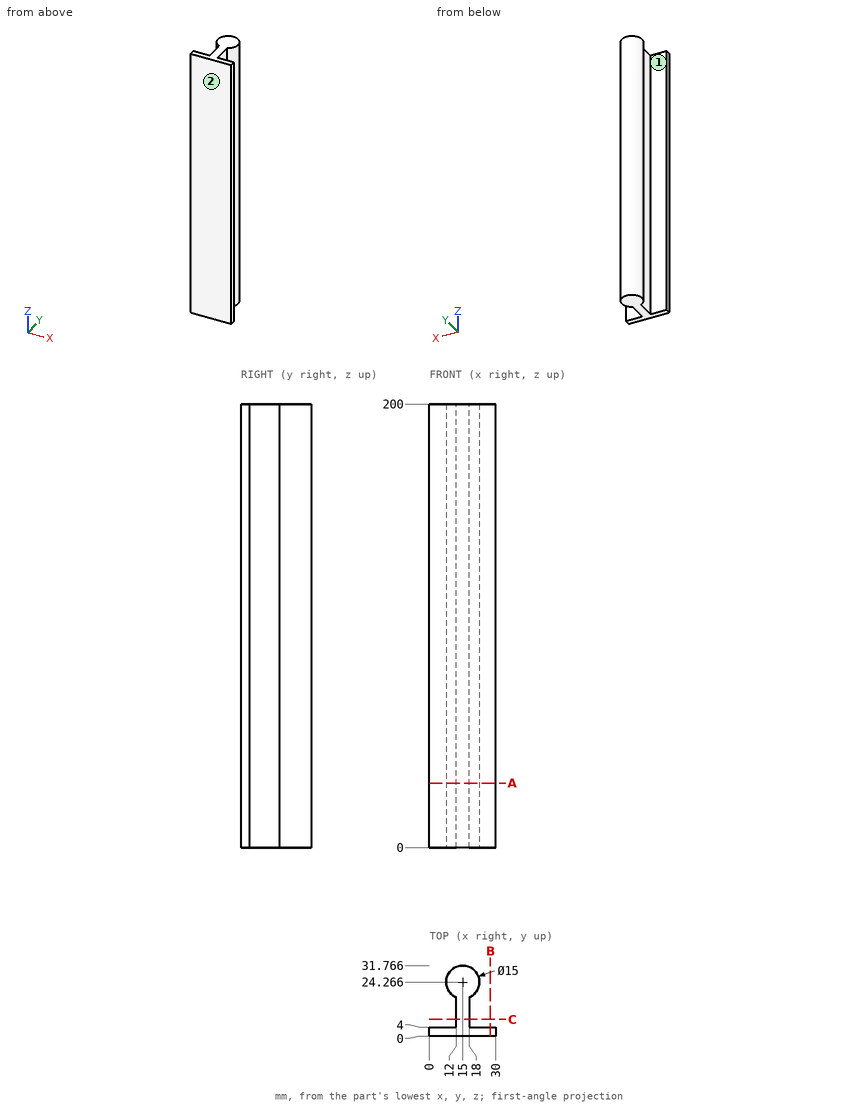
Check sheet for the drawn part. Datum: minimum x, y, z corner. Units: mm. Round coordinates to 2 decimals unless told otherwise and drop trailing zeros. Loops run counter-clockwise (first coordinate to the right, second up) from the corner with the lowest first, then second, coordinate; pieces in that order, holes last.
Item 1: Cross-section at A-A on z = 29. Record the boundary of the cut face in (x, y).
Item 2: Mould release check, pull along Y, two halves, no side actions. Record for the marked faces 1 and 2: pulls with the +Y half, pulls with the -Y half, needs draft (parallel to the pull), parting line crosses it, or undercut.
Item 3: Cross-section at C-C on y = 7.5. Record the boundary of the cut face in (x, z), then the cut area to 3 significant figures.
Item 4: Cross-section at B-B on x = 27.5. Record the boundary of the cut face in (y, z), then the cut area to 3 significant figures.
Item 5: Thickness scan on line 1 (X direction, y = 5, z = 40.5); line 2 (Y direction, x = 4.5, z = 97.5); line 3 (Y direction, x = 10.75, z = 165.5) (1 decimal). Record the ranges inside material, lowest first.
Item 6: Gauge pin test, flat ends, axial feed: pin 1 (6 mm diameter, centred on y = 22, z = 60, fed in from +X); pin 2 (6.5 mm diameter, centred on y = 12.5, z = 96.5, fed in from -X); pin 3 (5 mm diameter, centred on y = 17.5, z = 141.5, fed in from +X); pin 4 (12 mm diameter, centred on x = 9, z = 178, fed in from +Y). Record the tip position at first contact, or that the pin passes through.
Answer sheet:
1. outline: (0, 0) - (30, 0) - (30, 4) - (18, 4) - (18, 17.39) arc R7.5 ccw (long way) to (12, 17.39) - (12, 4) - (0, 4) - close
2. face 1: undercut
2. face 2: pulls with the -Y half
3. outline: (12, 0) - (18, 0) - (18, 200) - (12, 200) - close
3. area: 1,200 mm2
4. outline: (0, 0) - (4, 0) - (4, 200) - (0, 200) - close
4. area: 800 mm2
5. line 1: x = 12 to 18
5. line 2: y = 0 to 4
5. line 3: y = 0 to 4, 18.1 to 30.4
6. pin 1: stops at x = 22.5
6. pin 2: stops at x = 12
6. pin 3: stops at x = 21.17
6. pin 4: stops at y = 31.77
